Autodesk Inventor part; units mm, degrees
ref_plane "YZ Plane" through (0, 0, 0) normal (1, 0, 0) x (0, 1, 0)
ref_plane "XZ Plane" through (0, 0, 0) normal (0, 1, 0) x (-1, 0, 0)
ref_plane "XY Plane" through (0, 0, 0) normal (0, 0, 1) x (1, 0, 0)
sketch "Szkic1" plane through (0, 0, 0) normal (0, 1, 0) x (-1, 0, 0)
  line L0 (1.25, 50) -> (-1.25, 50)
  line L1 (-11.25, 40) -> (-11.25, -40)
  line L2 (-1.25, -50) -> (1.25, -50)
  line L3 (11.25, -40) -> (11.25, 40)
  line L4 (11.25, 50) -> (-11.25, -50)
  line L5 (11.25, -50) -> (-11.25, 50)
  arc A0 (11.25, 40) -> (1.25, 50) centre (1.25, 40) ccw
  arc A1 (-1.25, 50) -> (-11.25, 40) centre (-1.25, 40) ccw
  arc A2 (1.25, -50) -> (11.25, -40) centre (1.25, -40) ccw
  arc A3 (-11.25, -40) -> (-1.25, -50) centre (-1.25, -40) ccw
  point P0 (0, 0)
  point P1 (0, 0)
  dimension "d0" = 22.5
  dimension "d1" = 100
  dimension "d2" = 10
extrude "Wyciągnięcie proste1" add sketch "Szkic1" along normal blind 4.1
sketch "Szkic2" plane through (0, 4.1, 0) normal (0, 1, 0) x (1, 0, 0)
  circle A0 centre (0, 44) radius 3.5
  line L0 (1.25, 50) -> (-1.25, 50)
  point P0 (0, 0)
  point P1 (0, 50)
  dimension "d5" = 7
  dimension "d14" = 6
extrude "Wyciągnięcie proste2" cut sketch "Szkic2" against normal blind 8
sketch "Szkic3" plane through (0, 4.1, 0) normal (0, 1, 0) x (1, 0, 0)
  line L0 (0, 47.5) -> (0, 28.5)
  arc A0 (-2, 28.5) -> (2, 28.5) centre (0, 28.5) ccw
  line L1 (-2.75, 41.8349) -> (0, 41.8349)
  line L2 (1.25, 50) -> (-1.25, 50)
  line L3 (-2, 28.5) -> (-2.75, 41.8349)
  line L4 (2, 28.5) -> (2.75, 41.8349)
  line L5 (0, 41.8349) -> (2.75, 41.8349)
  circle A1 centre (0, 44) radius 3.5
  point P0 (0, 0)
  point P1 (0, 50)
  dimension "d8" = 19
  dimension "d10" = 5.5
  dimension "d22" = 13.3349
extrude "Wyciągnięcie proste3" cut sketch "Szkic3" against normal blind 1.1 contours L5 A1 L0 | L0 A1 L1 | A1 L4 A0 L3 picked at (1.6483, 41.6479) picked at (-1.6483, 41.6479)
sketch "Szkic4" plane through (0, 4.1, 0) normal (0, 1, 0) x (1, 0, 0)
  circle A0 centre (0, -44) radius 3.5
  line L0 (-1.25, -50) -> (1.25, -50)
  point P0 (0, 0)
  point P1 (0, -50)
  dimension "d15" = 7
  dimension "d16" = 6
extrude "Wyciągnięcie proste4" cut sketch "Szkic4" against normal blind 10
sketch "Szkic7" plane through (0, 4.1, 0) normal (0, 1, 0) x (1, 0, 0)
  line L0 (-1.25, -50) -> (1.25, -50)
  line L1 (0, -50) -> (0, -28.5)
  line L2 (0, -50) -> (0, -41.835)
  line L3 (0, -28.5) -> (0, -41.835)
  circle A0 centre (0, -44) radius 3.5
  line L4 (-2.75, -41.835) -> (2.75, -41.835)
  line L5 (-2.75, -41.835) -> (-2, -28.5)
  line L6 (2.75, -41.835) -> (1.9969, -28.3882)
  arc A1 (1.9969, -28.3882) -> (-2, -28.5) centre (0, -28.5) ccw
  point P0 (0, 0)
  dimension "d19" = 21.5
  dimension "d24" = 13.335
  dimension "d25" = 5.5001
extrude "Wyciągnięcie proste5" cut sketch "Szkic7" against normal blind 1.1 contours L5 A1 L6 A0
properties part number "arm_big_part"
Source: CAD feature listing. Evaluate the final solid. Frame: model axes, mm. A direction names the side the tool comes from. Round coordinates to 2 decimals unless told otherwise and drop trailing zeros. Loops run counter-clockwise (first coordinate to the right, second up) from the corner with the lowest first, then second, coordinate; pieces in that order, holes last.
(1) Contact query for flat-ended pins moving along their axis: pin 1 Ø1 at (x, y) = (4.5, 3.5) entering from -Z; pin 2 Ø3 at (x, z) = (0, 32) entering from +Y. Output: stop coordinate, or through.
From the geometry:
pin 1: stops at z = -49.61
pin 2: stops at y = 3
(2) Section query D-D (x = 9.75). Output: boundary loops of the cut face in (y, z), and give its area (3 significant figures).
From the geometry:
outline: (0, -45.27) - (4.1, -45.27) - (4.1, 45.27) - (0, 45.27) - close
area: 371 mm2
(3) Material intervals for probe 1 along Z at (x, y) = (0, 2.25); probe 2 along Z at (x, y) = (0.5, 3.95); probe 3 along Y at (x, z) = (-0.75, 32.5), sorted ascending.
From the geometry:
probe 1: z = -50 to -47.5, -40.5 to 40.5, 47.5 to 50
probe 2: z = -50 to -47.46, -26.56 to 26.56, 47.46 to 50
probe 3: y = 0 to 3
(4) Section query C-C (z = 44). Output: boundary loops of the cut face in (x, y).
From the geometry:
outline: (-10.42, 0) - (-3.5, 0) - (-3.5, 4.1) - (-10.42, 4.1) - close; (3.5, 0) - (10.42, 0) - (10.42, 4.1) - (3.5, 4.1) - close
(5) Access query for faces 1 (the cylindrical face through (8.4, 2.02, 46.99)), 2 (the flat face through (0, 3, 34)). Directions: +Z, -Z, +X, -X, +Y, -Y. A direction counts if a zero-diameter tool reaches every point of the face in a straight line with its end or side. Return the directions, or none.
From the geometry:
face 1: +Z, +X, +Y, -Y
face 2: +Y
(6) Section query B-B (y = 1.9). Output: boundary loops of the cut face in (x, z), and give its area (3 significant figures).
From the geometry:
outline: (-11.25, -40) arc R10 ccw to (-1.25, -50) - (1.25, -50) arc R10 ccw to (11.25, -40) - (11.25, 40) arc R10 ccw to (1.25, 50) - (-1.25, 50) arc R10 ccw to (-11.25, 40) - close; hole circle Ø7 at (0, -44); hole circle Ø7 at (0, 44)
area: 2,090 mm2
(7) Section query A-A (x = 0). Output: boundary loops of the cut face in (y, z), and give its area (3 significant figures).
From the geometry:
outline: (0, -50) - (4.1, -50) - (4.1, -47.5) - (0, -47.5) - close; (0, -40.5) - (3, -40.5) - (3, -26.5) - (4.1, -26.5) - (4.1, 26.5) - (3, 26.5) - (3, 40.5) - (0, 40.5) - close; (0, 47.5) - (4.1, 47.5) - (4.1, 50) - (0, 50) - close
area: 322 mm2
(8) Pull-direction query (X, two-part tool) for faces 3 (the flat face through (11.25, 2, 1)), 4 (the flat face through (0, 3, -34)), 5 (the cylindrical face through (0, 3.6, 26.5)), 6 (the cylindrical face through (-8.24, 2.02, 47.15)); classes: +X half, -X half, draft (parallel to the pull), parting line (faces both ways), or undercut.
From the geometry:
face 3: +X half
face 4: undercut
face 5: undercut
face 6: -X half
